```python
from build123d import *

# Parameters (mm, degrees)
SHAPE_BASE_R                   = 4.025
BOSS_EXTRUDE1_DEPTH            = 5
SWEEP2_START                   = -7.5
SWEEP2_DEPTH                   = 15
CUT_EXTRUDE2_REACH             = 52.965
BOSS_EXTRUDE2_DEPTH            = 15
CUT_EXTRUDE3_REACH             = 56.593
SKETCH4_10_R                   = 4.025
CUT_EXTRUDE3_DIRECTION_2_DEPTH = 55.593173935
FILLET1_R                      = 3
SKETCH21_W                     = 8
SKETCH21_H                     = 15
CUT_EXTRUDE4_DEPTH             = 2.5
F_6_CLEARANCE_HOLE1_D          = 4.3053
F_6_CLEARANCE_HOLE1_DEPTH      = 2.329629131


# Read off the part's stored shape, not the designer's step: Sweep2
with BuildPart() as part:
    # Shape - base → Boss-Extrude1 (new body)
    # profile 1 of 2: a face of its own
    with BuildSketch(Plane.XY):
        with BuildLine():
            Line((-10, 7.5), (25, 7.5))
            Line((25, 7.5), (25, -7.5))
            Line((25, -7.5), (-10, -7.5))
            ThreePointArc((-10, -7.5), (-13.535533906, -6.035533906), (-15, -2.5))
            Line((-15, -2.5), (-15, 2.5))
            ThreePointArc((-15, 2.5), (-13.535533906, 6.035533906), (-10, 7.5))
        make_face()
        Circle(SHAPE_BASE_R, mode=Mode.SUBTRACT)
    # profile 2 of 2: a face of its own
    with BuildSketch(Plane.XY):
        Circle(SHAPE_BASE_R)
    extrude(amount=-BOSS_EXTRUDE1_DEPTH)

    # Sweep2 outline → Sweep2 (add)
    with BuildSketch(Plane(origin=(0, 0, 0), x_dir=(1, 0, 0), z_dir=(0, 1, 0)).offset(SWEEP2_START)):
        Polygon((42.585185434, -6.869503049), (42.585185434, -11.147047613), (47.414814566, -9.852952387), (47.414814566, -4.130496951), (37.95038024, 1.529956073), (25, 5), (25, 0), (36.04961976, -2.960736691), align=None)
    extrude(amount=SWEEP2_DEPTH)

    # Sketch18 → Cut-Extrude2 (cut, up to next)
    with BuildSketch(Plane(origin=(0, 7.5, 0), x_dir=(1, 0, 0), z_dir=(0, 1, 0)), mode=Mode.PRIVATE) as cut_extrude2_sk1:
        Polygon((42.585185434, -11.147047613), (45, -10.5), (42.585185434, -10.5), align=None)
    cut_extrude2_tool1 = extrude(cut_extrude2_sk1.sketch, amount=-CUT_EXTRUDE2_REACH, mode=Mode.PRIVATE) & part.part
    add(cut_extrude2_tool1.solids().sort_by_distance((43.390124, 7.5, 10.715683))[0], mode=Mode.SUBTRACT)

    # Sketch18<3> → Boss-Extrude2 (add, through all)
    with BuildSketch(Plane(origin=(0, 7.5, 0), x_dir=(1, 0, 0), z_dir=(0, 1, 0))):
        Polygon((47.414814566, -10.5), (47.414814566, -9.852952387), (45, -10.5), align=None)
    extrude(amount=-BOSS_EXTRUDE2_DEPTH)

    # Mirror1: part across face


with BuildPart() as part_1:
    add(part.part)
    add(part.part.mirror(Plane(origin=(45, 0, 10.5), x_dir=(1, 0, 0), z_dir=(0, 0, 1))))

    # Sketch4<10> → Cut-Extrude3 (cut, up to next)
    with BuildSketch(Plane.XY, mode=Mode.PRIVATE) as cut_extrude3_sk1:
        with Locations(Location((0, 0, 0), (0, 0, 180))):
            Circle(SKETCH4_10_R)
    cut_extrude3_tool1 = extrude(cut_extrude3_sk1.sketch, amount=-CUT_EXTRUDE3_REACH, mode=Mode.PRIVATE) & part_1.part
    add(cut_extrude3_tool1.solids().sort_by_distance((0, 0, 0))[0], mode=Mode.SUBTRACT)

    # Sketch4<10> → Cut-Extrude3 direction 2 (cut)
    with BuildSketch(Plane.XY):
        with Locations(Location((0, 0, 0), (0, 0, 180))):
            Circle(SKETCH4_10_R)
    extrude(amount=CUT_EXTRUDE3_DIRECTION_2_DEPTH, mode=Mode.SUBTRACT)

    # Fillet1
    fillet1_edges = [part_1.edges().sort_by_distance(p)[0] for p in [
        (47.414814566, 0, 4.130496951),
        (42.585185434, 0, 6.869503049),
        (37.95038024, 0, -1.529956073),
        (36.04961976, 0, 2.960736691),
        (25, 0, -5),
        (25, 0, 0),
        (25, 0, 21),
        (42.585185434, 0, 14.130496951),
        (47.414814566, 0, 16.869503049),
        (37.95038024, 0, 22.529956073),
        (36.04961976, 0, 18.039263309),
        (25, 0, 26),
    ]]
    fillet(fillet1_edges, radius=FILLET1_R)

    # Sketch21 → Cut-Extrude4 (cut)
    with BuildSketch(Plane(origin=(47.414814566, 0, 0), x_dir=(0, 0, -1), z_dir=(1, 0, 0))):
        with Locations((-10.5, 0)):
            Rectangle(SKETCH21_W, SKETCH21_H)
    extrude(amount=-CUT_EXTRUDE4_DEPTH, mode=Mode.SUBTRACT)

    # #6 Clearance Hole1
    with Locations(Plane(origin=(44.914814566, 0, 0), x_dir=(0, 0, -1), z_dir=(1, 0, 0))):
        with Locations((-10.5, 0)):
            Hole(F_6_CLEARANCE_HOLE1_D / 2, depth=F_6_CLEARANCE_HOLE1_DEPTH)


solid = part_1.part
```
For this review, take the finished solid that the model builds, in its own axes (mm). A direction names the side the tool comes from. Round coordinates to 2 decimals unless told otherwise and drop trailing zeros. Write each loop counter-clockwise with the first axis right and the second up, starting at its lowest first coordinate (ties: lowest second). Pieces come first, ordered by that corner, then holes. Notation, with made-up numbers: (59, 26.25) - (99, 26.25) arc R27 ccw to (99, 61.25) - close; hole circle Ø4 at (33, -23). An arc over 180 degrees is marked (long way). Answer as a JSON object with one key per item and string values.
1. Tool access review of faces 4 (the face through (42.585, 5, 11)), 5 (the face through (46, 0, 14.5)), 6 (the face through (31.549, -0.105, -3.245)): name each direction out of +Z, -Z, +X, -X, +Y, -Y from which nothing blocks a thin tool from reaching the whole face with its end or side.
Response values:
{"face 4": "-X, +Y, -Y", "face 5": "+X, +Y, -Y", "face 6": "-Z, +X, +Y, -Y"}
2. Draft analysis for pull direction Y (two halves, no side actions). For faces 1 (the face through (-3.84, -1.21, 23.46)), 2 (the face through (42.2, 0.1, 13.9)), 3 (the face through (-13.57, 6, 23.46)), state which applies: +Y half, -Y half, draft (parallel to the pull), parting line (faces both ways), or undercut.
Response values:
{"face 1": "undercut", "face 2": "draft", "face 3": "+Y half"}
3. We need section B-B on x = 0. Give the boundary of the cut face in (y, z) (3 decimals).
Response values:
{"outline": "(-7.5, -5) - (-4.025, -5) - (-4.025, 0) - (-7.5, 0) - close; (-7.5, 21) - (-4.025, 21) - (-4.025, 26) - (-7.5, 26) - close; (4.025, -5) - (7.5, -5) - (7.5, 0) - (4.025, 0) - close; (4.025, 21) - (7.5, 21) - (7.5, 26) - (4.025, 26) - close"}
4. We need section A-A on z = 10.5. Give the boundary of the cut face in (x, y).
Response values:
{"outline": "(42.59, -7.5) - (44.91, -7.5) - (44.91, -2.15) - (42.59, -2.15) - close; (42.59, 2.15) - (44.91, 2.15) - (44.91, 7.5) - (42.59, 7.5) - close"}
5. For pin 1 Ø1 at (x, y) = (28.5, -3.5) entering from -Z; pin 2 Ø8 at (y, z) = (-6, 19.5) entering from -X; pin 3 Ø4 at (y, z) = (-2, 11.5) entering from +X; pin 4 Ø2 at (x, y) = (46, -3.5) entering from +Z, all flat-tipped, find the tip position at first contact; note any pin that passes through.
Response values:
{"pin 1": "stops at z = -4.2", "pin 2": "stops at x = -15", "pin 3": "stops at x = 44.91", "pin 4": "stops at z = 18.31"}
6. We need section C-C on x = 30. Give the boundary of the cut face in (y, z).
Response values:
{"outline": "(-7.5, -3.66) - (7.5, -3.66) - (7.5, 1.34) - (-7.5, 1.34) - close; (-7.5, 19.66) - (7.5, 19.66) - (7.5, 24.66) - (-7.5, 24.66) - close"}
7. We need section D-D on y = 0. Count the separate pieces of the cut face and the enclosed holes in it, then the cut area to 3 significant figures.
Response values:
{"separate pieces": "4", "enclosed holes": "0", "area": "548 mm2"}
8. To check wall thickness, follow line 1 along Y through (x, z) = (44.05, 10.5); line 2 along Z through (x, y) = (-4, -2); line 3 along Y through (x, z) = (0, -2) (3 decimals). State the ranges of each line that lie inside material, in increasing order.
Response values:
{"line 1": "y = -7.5 to -2.15, 2.15 to 7.5", "line 2": "z = -5 to 0, 21 to 26", "line 3": "y = -7.5 to -4.025, 4.025 to 7.5"}
